from build123d import *

# Parameters (mm, degrees)
F0_W     = 76.2
F0_H     = 12.7
F1_DEPTH = 5.334
F3_DEPTH = 12.7
F4_R     = 3.8
F5_DEPTH = 1


with BuildPart() as f1:
    # F0 (on Top) → F1 (new body)
    with BuildSketch(Plane.XY):
        with Locations((-2.639927, -2.647982)):
            Rectangle(F0_W, F0_H)
    extrude(amount=F1_DEPTH)

    # F2 (on face) → F3 (join, through all)
    with BuildSketch(Plane.XZ.offset(8.997982)):
        Polygon((-40.739927, 5.334), (-37.917357, 5.334), (-35.98541, 8.101238), (-40.739927, 8.101238), align=None)
        Polygon((30.705556, 8.101238), (32.637503, 5.334), (35.460073, 5.334), (35.460073, 8.101238), align=None)
    extrude(amount=-F3_DEPTH)

    # F4 (on face) → F5 (cut)
    with BuildSketch(Plane(origin=(0, 0, 0), x_dir=(1, 0, 0), z_dir=(0, 0, -1))):
        with Locations((-31.556085, 2.647982)):
            Circle(F4_R)
        with Locations((26.276231, 2.647982)):
            Circle(F4_R)
    extrude(amount=-F5_DEPTH, mode=Mode.SUBTRACT)


solid = f1.part
Here's how the part is built. I have some questions about the finished solid (model axes, mm). A direction names the side the tool comes from. Coordinates: 2 decimals unless noted, no trailing zeros. Write each loop counter-clockwise with the first axis right and the second up, starting at its lowest first coordinate (ties: lowest second). Pieces come first, ordered by that corner, then holes.
Item 1: Will this pin go through, and if not, where does the flat tip stop? pin 1 (5 mm diameter, centred on x = 27.5, y = 1.5, fed in from +Z).
Item 2: If I drill on line 1 (Z direction, x = 2.5, y = 0.5); line 2 (X direction, y = -2.5, z = 7.5); line 3 (Z direction, x = -32, y = -3.5), over which ranges is the centre line in solid material (lowest first)?
Item 3: If we mould it in two halves opening along X, with no side actions, what happens to faces 4 (the flat face through (35.46, -3, 4)), 5 (the flat face through (-3, -8.998, 3)), 6 (the flat face through (26, -3, 1)), 7 (the flat face through (-40.74, -3, 4))? For each: +X half, -X half, draft (parallel to the pull), parting line (faces both ways), or undercut.
Item 4: I want a section at A-A on y = -4. Write out the boundary of the cut face in (x, z).
Item 5: On a 3-axis mill with a long thin cutter (end or side, diameter ignored), from which of +Z, -Z, +X, -X, +Y, -Y can I reach the whole of each face in a straight line? I mean faces 1 (the cylindrical face through (28.03, 0.723, 0.493)), 2 (the flat face through (-38, -3, 8.101)), 3 (the flat face through (-36.965, -2.737, 6.698)). Say none if no direction works.
Item 6: I want a section at B-B on x = -28.5. Write out the boundary of the cut face in (y, z), and give its area (3 significant figures).
Item 7: I want a section at C-C on y = -0.25. Write out the boundary of the cut face in (x, z).
Item 8: I want a section at D-D on x = 26. Write out the boundary of the cut face in (y, z), and give its area (3 significant figures).
Findings below:
1. pin 1: stops at z = 5.33
2. line 1: z = 0 to 5.33
2. line 2: x = -40.74 to -36.41, 31.13 to 35.46
2. line 3: z = 1 to 5.33
3. face 4: +X half
3. face 5: draft
3. face 6: undercut
3. face 7: -X half
4. outline: (-40.74, 0) - (-35.11, 0) - (-35.11, 1) - (-28, 1) - (-28, 0) - (22.72, 0) - (22.72, 1) - (29.83, 1) - (29.83, 0) - (35.46, 0) - (35.46, 8.1) - (30.71, 8.1) - (32.64, 5.33) - (-37.92, 5.33) - (-35.99, 8.1) - (-40.74, 8.1) - close
5. face 1: -Z
5. face 2: +Z, +X, -X, +Y, -Y
5. face 3: +Y, -Y
6. outline: (-9, 0) - (-4.91, 0) - (-4.91, 1) - (-0.39, 1) - (-0.39, 0) - (3.7, 0) - (3.7, 5.33) - (-9, 5.33) - close
6. area: 63.2 mm2
7. outline: (-40.74, 0) - (-34.5, 0) - (-34.5, 1) - (-28.61, 1) - (-28.61, 0) - (23.33, 0) - (23.33, 1) - (29.22, 1) - (29.22, 0) - (35.46, 0) - (35.46, 8.1) - (30.71, 8.1) - (32.64, 5.33) - (-37.92, 5.33) - (-35.99, 8.1) - (-40.74, 8.1) - close
8. outline: (-9, 0) - (-6.44, 0) - (-6.44, 1) - (1.14, 1) - (1.14, 0) - (3.7, 0) - (3.7, 5.33) - (-9, 5.33) - close
8. area: 60.2 mm2
